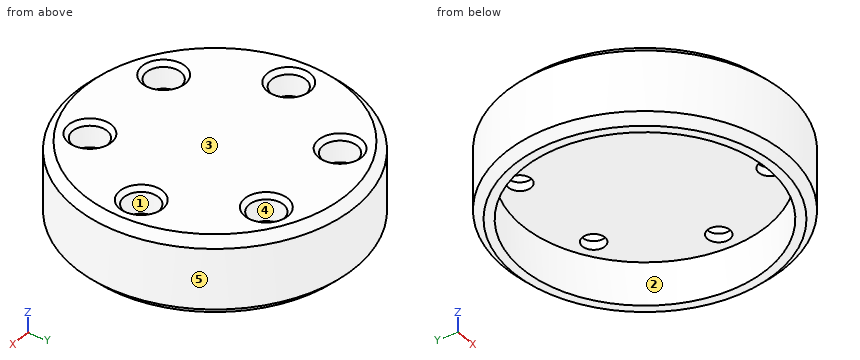
```python
from build123d import *

# Parameters (mm, degrees)
SKETCH_1_R                           = 32.5
EXTRUDE_1_DEPTH                      = 9
CHAMFER_1_SIZE                       = 2
SKETCH_3_R                           = 2.6
CUT_EXTRUDE_1_DEPTH                  = 47.834816109
CUT_EXTRUDE_START                    = 9
SKETCH_4_R                           = 4
CUT_EXTRUDE_2_DEPTH                  = 6
CHAMFER_2_SIZE                       = 1
PATTERN_CIRCULAR_1_COUNT             = 6
CHAMFER_2_OF_PATTERN_CIRCULAR_1_SIZE = 1
SKETCH_5_R                           = 28.4
CUT_EXTRUDE_3_DEPTH                  = 10


with BuildPart() as part:
    # ｽｹｯﾁ1 → ﾎﾞｽ - 押し出し1 (new, symmetric)
    with BuildSketch(Plane.XY):
        Circle(SKETCH_1_R)
    extrude(amount=EXTRUDE_1_DEPTH, both=True)

    # 面取り1
    chamfer_1_edges = [part.edges().sort_by_distance(p)[0] for p in [
        (-32.5, 0, -9),
        (-32.5, 0, 9),
    ]]
    chamfer(chamfer_1_edges, length=CHAMFER_1_SIZE)

    # ｽｹｯﾁ3 → ｶｯﾄ - 押し出し1 (cut, symmetric)
    with BuildSketch(Plane.XY):
        with Locations((11.875, 20.56810334)):
            Circle(SKETCH_3_R)
    cut_extrude_1 = extrude(amount=CUT_EXTRUDE_1_DEPTH, both=True, mode=Mode.SUBTRACT)

    # ｽｹｯﾁ4 → ｶｯﾄ - 押し出し2 (cut)
    with BuildSketch(Plane.XY.offset(CUT_EXTRUDE_START)):
        with Locations((11.875, 20.56810334)):
            Circle(SKETCH_4_R)
    cut_extrude_2 = extrude(amount=-CUT_EXTRUDE_2_DEPTH, mode=Mode.SUBTRACT)

    # 面取り2
    chamfer_2_edges = [part.edges().sort_by_distance(p)[0] for p in [
        (7.875, 20.56810334, 9),
    ]]
    chamfer(chamfer_2_edges, length=CHAMFER_2_SIZE)

    # 円形ﾊﾟﾀｰﾝ1: ｶｯﾄ - 押し出し1, ｶｯﾄ - 押し出し2 ×6 about axis
    pattern_circular_1_axis = Axis((0, 0, 0), (0, 0, 1))
    add([cut_extrude_1.rotate(pattern_circular_1_axis, i * 360 / PATTERN_CIRCULAR_1_COUNT) for i in range(1, PATTERN_CIRCULAR_1_COUNT)], mode=Mode.SUBTRACT)
    add([cut_extrude_2.rotate(pattern_circular_1_axis, i * 360 / PATTERN_CIRCULAR_1_COUNT) for i in range(1, PATTERN_CIRCULAR_1_COUNT)], mode=Mode.SUBTRACT)

    # 面取り2 of 円形ﾊﾟﾀｰﾝ1
    chamfer_2_of_pattern_circular_1_edges = [part.edges().sort_by_distance(p)[0] for p in [
        (-13.875, 17.104001725, 9),
        (-21.75, -3.464101615, 9),
        (-7.875, -20.56810334, 9),
        (13.875, -17.104001725, 9),
        (21.75, 3.464101615, 9),
    ]]
    chamfer(chamfer_2_of_pattern_circular_1_edges, length=CHAMFER_2_OF_PATTERN_CIRCULAR_1_SIZE)

    # ｽｹｯﾁ5 → ｶｯﾄ - 押し出し3 (cut)
    with BuildSketch(Plane(origin=(0, 0, -9), x_dir=(-1, 0, 0), z_dir=(0, 0, -1))):
        Circle(SKETCH_5_R)
    extrude(amount=-CUT_EXTRUDE_3_DEPTH, mode=Mode.SUBTRACT)


solid = part.part
```
Can you work these out from the model? Positions are in its coordinate system, mm. Face numbers are marked on the shaded views. A direction names the side the tool comes from. Round coordinates to 2 decimals unless told otherwise and drop trailing zeros. Loops run counter-clockwise (first coordinate to the right, second up) from the corner with the lowest first, then second, coordinate; pieces in that order, holes last. Notation, with made-up numbers: M 48.5,-21 L 52.5,-21 A28 ccw 52.5,6 Z; hole C 80,-8 d3. An arc over 180 degrees is marked long. Answer as a JSON object with one key per item and string values. Group by question number.
Q1. On a 3-axis mill with a long thin cutter (end or side, diameter ignored), from which of +Z, -Z, +X, -X, +Y, -Y can I reach the whole of each face in a straight line? I mean the marked faces 1 and 2. Say none if no direction works.
Q2. Will these pins go through, and if not, where does the flat tip stop? pin 1 (7 mm diameter, centred on x = -11.88, y = -20.57, fed in from -Z); pin 2 (4 mm diameter, centred on x = -23.75, y = 0, fed in from -Z); pin 3 (7 mm diameter, centred on x = 11.88, y = 20.57, fed in from +Z); pin 4 (4 mm diameter, centred on x = 8.5, z = 5.5, fed in from +Y).
Q3. Please list where these lines run through material, in increasing order: L1, parallel to Y at x = 14, z = 4.75; L2, parallel to Z at x = 6, y = 21; L3, parallel to X at y = -17, z = 5.75.
Q4. Imagine slicing it at A-A, the plane y = 0. Count the separate pieces of the cut face and the enclosed holes in it, then the cut area to 3 significant figures.
Q5. Imagine slicing it at C-C, the plane z = 0.25. Please give me the cut outline in (x, y).
Q6. Imagine slicing it at B-B, the plane x = 0. Please give me the cut outline in (y, z), then the cut area to 3 significant figures.
Q7. We'd pull the mould along Y, two halves only. Please class the marked faces 3, 4 and 5: +Y half, -Y half, draft (parallel to the pull), parting line (faces both ways), or undercut.
Findings:
{
 "1": {"face 1": "+Z", "face 2": "-Z"},
 "2": {"pin 1": "stops at z = 1", "pin 2": "passes through", "pin 3": "stops at z = 3", "pin 4": "stops at y = 31.84"},
 "3": {"L1": "y = -29.33 to -23.96, -17.18 to 17.18, 23.96 to 29.33", "L2": "z = 1 to 9", "L3": "x = -27.7 to -13.68, -10.07 to 10.07, 13.68 to 27.7"},
 "4": {"separate pieces": "3", "enclosed holes": "0", "area": "475 mm2"},
 "5": {"outline": "C 0,0 d65; hole C 0,0 d56.8"},
 "6": {"outline": "M -32.5,-7 L -30.5,-9 L -28.4,-9 L -28.4,1 L 28.4,1 L 28.4,-9 L 30.5,-9 L 32.5,-7 L 32.5,7 L 30.5,9 L -30.5,9 L -32.5,7 Z", "area": "594 mm2"},
 "7": {"face 3": "draft", "face 4": "undercut", "face 5": "parting line"}
}
